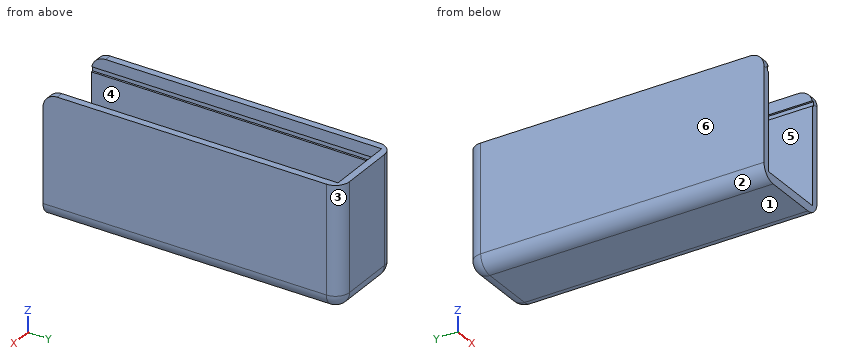
from build123d import *

# Parameters (mm, degrees)
F1_DEPTH = 40
F0_W     = 24
F0_H     = 100
F0_H_2   = 2.5
F2_DEPTH = 3
F3_W     = 0.7
F3_H     = 1.8
F4_DEPTH = 102.5
F5_R     = 5


with BuildPart() as f1:
    # F0 (on Top) → F1 (new body)
    with BuildSketch(Plane.XY):
        Polygon((12, 50), (12, -50), (12, -52.5), (14.5, -52.5), (14.5, 52.5), (-14.5, 52.5), (-14.5, -52.5), (-12, -52.5), (-12, -50), (-12, 50), align=None)
    extrude(amount=F1_DEPTH)

    # F0 (on Top) → F2 (join)
    with BuildSketch(Plane.XY):
        Rectangle(F0_W, F0_H)
        Polygon((12, 50), (12, -50), (12, -52.5), (14.5, -52.5), (14.5, 52.5), (-14.5, 52.5), (-14.5, -52.5), (-12, -52.5), (-12, -50), (-12, 50), align=None)
        with Locations((0, -51.25)):
            Rectangle(F0_W, F0_H_2)
    extrude(amount=-F2_DEPTH)

    # F3 (on face) → F4 (cut)
    with BuildSketch(Plane.XZ.offset(52.5)):
        with Locations((-12.35, 35.1)):
            Rectangle(F3_W, F3_H)
        with Locations((12.35, 35.1)):
            Rectangle(F3_W, F3_H)
    extrude(amount=-F4_DEPTH, mode=Mode.SUBTRACT)

    # F5
    f5_edges = [f1.edges().sort_by_distance(p)[0] for p in [
        (-13.25, -52.5, 40),
        (13.25, -52.5, 40),
        (-14.5, 52.5, 18.5),
        (14.5, 52.5, 18.5),
        (0, 52.5, -3),
        (14.5, 0, -3),
        (-14.5, 0, -3),
    ]]
    fillet(f5_edges, radius=F5_R)


solid = f1.part
The model under review builds one solid part; all positions refer to its coordinate system, in mm. Face numbers are marked on the shaded views. A direction names the side the tool comes from. Round coordinates to 2 decimals unless told otherwise and drop trailing zeros. Write each loop counter-clockwise with the first axis right and the second up, starting at its lowest first coordinate (ties: lowest second). Pieces come first, ordered by that corner, then holes. Notation, with made-up numbers: M 71.5,37 L 102.5,37 A10 ccw 102.5,48 Z; hole C 89,72.5 d9. An arc over 180 degrees is marked long. Use a Markdown table: item, result. Add a question column.
Q1. We need section A-A, the plane x = -4.5. State the section outline as (y, z) points.
Q2. The part is to be moulded in two halves that separate along X. For the marked faces 1, 2, 3 and 4, say which applies: pulls with the +X half, pulls with the -X half, needs draft (parallel to the pull), parting line crosses it, or undercut.
Q3. We need section D-D, the plane x = 10.5. State the section outline as (y, z) points, plus the area to 3 significant figures.
Q4. Insertion check: pin 1 (1 mm diameter, centred on x = 5.5, z = 30.5, fed in from -Y); pin 2 (12 mm diameter, centred on x = 11.5, z = 32.5, fed in from -Y); pin 3 (1 mm diameter, centred on x = -0.5, y = 32.5, fed in from +Z). Each pin has a flat end and moves straight along its axis. Give the tip position at first contact, or say it passes through.
Q5. We need section C-C, the plane y = 42. State the section outline as (x, z) points, plus the area to 3 significant figures.
Q6. We need section B-B, the plane z = 7.5. State the section outline as (x, y) points, plus the area to 3 significant figures.
Q7. Machinability: for the marked faces 5 and 6, which of the approach directions +Z, -Z, +X, -X, +Y, -Y give a long, thin tool a straight path to every point of the face, cutting with its end or side? Answer none if there is none.
Q8. To check wall thickness, follow line 1 (X direction, y = 36, z = 24); line 2 (Z direction, x = -7.5, y = 17); line 3 (Y direction, x = -9.25, z = 9). State the ranges of each line that lie inside material, in increasing order.
Findings below:
| question | item | result |
|---|---|---|
| 1 | outline | M -52.5,-3 L 47.5,-3 A5 ccw 52.5,2 L 52.5,40 L 50,40 L 50,0 L -52.5,0 Z |
| 2 | face 1 | needs draft |
| 2 | face 2 | pulls with the -X half |
| 2 | face 3 | pulls with the +X half |
| 2 | face 4 | undercut |
| 3 | outline | M -52.5,-2.9 L 47.5,-2.9 A4.9 ccw 52.4,2 L 52.4,40 L 50,40 L 50,0 L -52.5,0 Z |
| 3 | area | 395 mm² |
| 4 | pin 1 | stops at y = 50 |
| 4 | pin 2 | stops at y = -52.5 |
| 4 | pin 3 | stops at z = 0 |
| 5 | outline | M -14.5,2 A5 ccw -9.5,-3 L 9.5,-3 A5 ccw 14.5,2 L 14.5,40 L 12,40 L 12,36 L 12.7,36 L 12.7,34.2 L 12,34.2 L 12,0 L -12,0 L -12,34.2 L -12.7,34.2 L -12.7,36 L -12,36 L -12,40 L -14.5,40 Z |
| 5 | area | 274 mm² |
| 6 | outline | M -14.5,-52.5 L -12,-52.5 L -12,50 L 12,50 L 12,-52.5 L 14.5,-52.5 L 14.5,47.5 A5 ccw 9.5,52.5 L -9.5,52.5 A5 ccw -14.5,47.5 Z |
| 6 | area | 574 mm² |
| 7 | face 5 | +Z, -Y |
| 7 | face 6 | +Z, -Z, -X, +Y, -Y |
| 8 | line 1 | x = -14.5 to -12, 12 to 14.5 |
| 8 | line 2 | z = -3 to 0 |
| 8 | line 3 | y = 50 to 52.5 |
